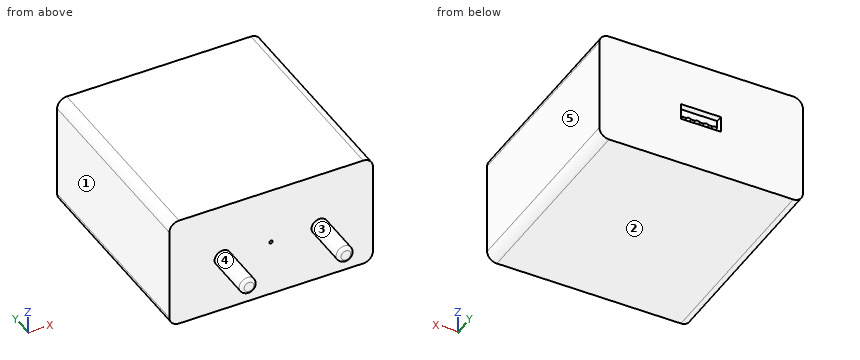
```python
from build123d import *

# Parameters (mm, degrees)
SKETCH1_W           = 63
SKETCH1_H           = 35
BOSS_EXTRUDE1_DEPTH = 64
FILLET1_R           = 3
SKETCH2_R           = 2.5
BOSS_EXTRUDE2_DEPTH = 15
FILLET2_R           = 1
SKETCH4_R           = 0.5
CUT_EXTRUDE1_DEPTH  = 1
SKETCH5_W           = 12.3
SKETCH5_H           = 5
CUT_EXTRUDE2_DEPTH  = 13
BOSS_EXTRUDE3_DEPTH = 11


with BuildPart() as part:
    # Sketch1 → Boss-Extrude1 (new body)
    with BuildSketch(Plane(origin=(0, 0, 0), x_dir=(1, 0, 0), z_dir=(0, 1, 0))):
        Rectangle(SKETCH1_W, SKETCH1_H)
    extrude(amount=BOSS_EXTRUDE1_DEPTH)

    # Fillet1
    fillet1_edges = [part.edges().sort_by_distance(p)[0] for p in [
        (31.5, 32, 17.5),
        (-31.5, 32, 17.5),
        (-31.5, 32, -17.5),
        (31.5, 32, -17.5),
    ]]
    fillet(fillet1_edges, radius=FILLET1_R)

    # Sketch2 → Boss-Extrude2 (add)
    with BuildSketch(Plane.XZ):
        with Locations(Location((-15, 0, 0), (0, 0, 270))):
            Circle(SKETCH2_R)
        with Locations(Location((15, 0, 0), (0, 0, 90))):
            Circle(SKETCH2_R)
    extrude(amount=BOSS_EXTRUDE2_DEPTH)

    # Fillet2
    fillet2_edges = [part.edges().sort_by_distance(p)[0] for p in [
        (-15, -15, 2.5),
        (15, -15, -2.5),
    ]]
    fillet(fillet2_edges, radius=FILLET2_R)

    # Sketch4 → Cut-Extrude1 (cut)
    with BuildSketch(Plane.XZ):
        with Locations(Location((0, 0, 0), (0, 0, 270))):
            Circle(SKETCH4_R)
    extrude(amount=-CUT_EXTRUDE1_DEPTH, mode=Mode.SUBTRACT)

    # Sketch5 → Cut-Extrude2 (cut)
    with BuildSketch(Plane(origin=(0, 64, 0), x_dir=(1, 0, 0), z_dir=(0, 1, 0))):
        Rectangle(SKETCH5_W, SKETCH5_H)
    extrude(amount=-CUT_EXTRUDE2_DEPTH, mode=Mode.SUBTRACT)

    # Sketch6 → Boss-Extrude3 (add)
    with BuildSketch(Plane(origin=(0, 51, 0), x_dir=(1, 0, 0), z_dir=(0, 1, 0))):
        with BuildLine():
            Line((-6.07, -0.08), (-6.07, -2.42))
            Line((-6.07, -2.42), (6.07, -2.42))
            Line((6.07, -2.42), (6.07, -0.08))
            add(Edge.make_bspline(
                [(6.07, -0.08), (5.375982436, -0.656866539), (4.618995195, -0.08)],
                knots=[0.014708799, 0.014708799, 0.014708799, 0.930781283, 0.930781283, 0.930781283], degree=2))
            Line((4.618995195, -0.08), (3.421648134, -0.08))
            add(Edge.make_bspline(
                [(3.421648134, -0.08), (2.695459097, -0.701406982), (1.95, -0.08)],
                knots=[0.014708799, 0.014708799, 0.014708799, 0.984687043, 0.984687043, 0.984687043], degree=2))
            Line((1.95, -0.08), (0.721648134, -0.08))
            add(Edge.make_bspline(
                [(0.721648134, -0.08), (-0.004540903, -0.701406982), (-0.75, -0.08)],
                knots=[0.014708799, 0.014708799, 0.014708799, 0.984687043, 0.984687043, 0.984687043], degree=2))
            Line((-0.75, -0.08), (-1.978351866, -0.08))
            add(Edge.make_bspline(
                [(-1.978351866, -0.08), (-2.704540903, -0.701406982), (-3.45, -0.08)],
                knots=[0.014708799, 0.014708799, 0.014708799, 0.984687043, 0.984687043, 0.984687043], degree=2))
            Line((-3.45, -0.08), (-4.678351866, -0.08))
            add(Edge.make_bspline(
                [(-4.678351866, -0.08), (-5.393535509, -0.624780928), (-6.07, -0.08)],
                knots=[0.084890823, 0.084890823, 0.084890823, 0.984687043, 0.984687043, 0.984687043], degree=2))
        make_face()
    extrude(amount=BOSS_EXTRUDE3_DEPTH)


solid = part.part
```
The listing builds one solid part. Answer for the finished solid, in the listing's coordinates (mm). Face numbers are marked on the shaded views. A direction names the side the tool comes from. Give positions to 0.01 mm unless a question says otherwise; leave off trailing zeros. Order: outer loops, then holes, each group sorted by start corner. A loop starts at its lowest first (then second) coordinate and runs counter-clockwise, first axis right, second up. Notation, with made-up numbers: (-4.75, 74) -> (5.25, 74) arc R14 ccw to (5.25, 87) -> close; hole circle Ø10 at (69, -9). An arc over 180 degrees is marked (long way). Answer as CSV lines item,"result". Start each with the question number.
Q1. A cutting plane is placed at C-C (x = 23). Determine the outline of the cut face in (y, z), then the cut area to 3 significant figures.
Q2. Determine the mould class of the marked faces 1, 2 and 3 for opening direction X: pulls with the +X half, pulls with the -X half, needs draft (parallel to the pull), parting line crosses it, or undercut.
Q3. A cutting plane is placed at B-B (z = 6.5). Determine the outline of the cut face in (x, y).
Q4. Given pin 1 (8 mm diameter, centred on x = 9, z = 12.5, fed in from -Y); pin 2 (1.5 mm diameter, centred on x = 0.5, z = 0, fed in from +Y); pin 3 (0.5 mm diameter, centred on x = 0, z = 0, fed in from -Y), each flat-ended and moving along its own axis, determine where each tip first touches the part or whether it passes through.
Q5. Find the intervals of material crossed by L1, parallel to X at y = 0.65, z = 0; L2, parallel to Y at x = -5, z = -7; L3, parallel to X at y = 23, z = 15.5, in increasing order.
Q6. A cutting plane is placed at A-A (x = -15). Determine the outline of the cut face in (y, z).
Q7. Which of the six approach directions +Z, -Z, +X, -X, +Y, -Y give full straight-line access (tool end or side, diameter ignored) to the marked faces 4 and 5?
Results found:
1,outline,"(0, -17.5) -> (64, -17.5) -> (64, 17.5) -> (0, 17.5) -> close"
1,area,"2,240 mm2"
2,face 1,"pulls with the -X half"
2,face 2,"needs draft"
2,face 3,"undercut"
3,outline,"(-31.5, 0) -> (31.5, 0) -> (31.5, 64) -> (-31.5, 64) -> close"
4,pin 1,"y = 0"
4,pin 2,"y = 62"
4,pin 3,"y = 1"
5,L1,"-31.5 to -0.5, 0.5 to 31.5"
5,L2,"0 to 64"
5,L3,"-31.33 to 31.33"
6,outline,"(-15, -1.5) arc R1 ccw to (-14, -2.5) -> (0, -2.5) -> (0, -17.5) -> (64, -17.5) -> (64, 17.5) -> (0, 17.5) -> (0, 2.5) -> (-14, 2.5) arc R1 ccw to (-15, 1.5) -> close"
7,face 4,"-Y"
7,face 5,"+Z, -Z, +X, +Y, -Y"
